```python
from build123d import *

# Parameters (mm, degrees)
SKETCH1_R           = 0.75
SKETCH1_W           = 10.15
SKETCH1_H           = 5.15
BOSS_EXTRUDE1_DEPTH = 7
SKETCH2_W           = 13.15
SKETCH2_H           = 8.15
BOSS_EXTRUDE2_DEPTH = 2


with BuildPart() as part:
    # Sketch1 → Boss-Extrude1 (new body)
    with BuildSketch(Plane.XY):
        with BuildLine():
            Line((-6.58, 4.075), (-1.505, 4.075))
            Line((-1.505, 4.075), (-1.505, 5.575))
            ThreePointArc((-1.505, 5.575), (-0.005, 7.075), (1.495, 5.575))
            Line((1.495, 5.575), (1.495, 4.075))
            Line((1.495, 4.075), (6.57, 4.075))
            Line((6.57, 4.075), (6.57, -4.075))
            Line((6.57, -4.075), (-6.58, -4.075))
            Line((-6.58, -4.075), (-6.58, 4.075))
        make_face()
        with Locations((-0.005, 5.575)):
            Circle(SKETCH1_R, mode=Mode.SUBTRACT)
        with Locations((-0.005, 0)):
            Rectangle(SKETCH1_W, SKETCH1_H, mode=Mode.SUBTRACT)
    extrude(amount=BOSS_EXTRUDE1_DEPTH)

    # Sketch2 → Boss-Extrude2 (add)
    with BuildSketch(Plane.XY.offset(7)):
        with Locations((-0.005, 0)):
            Rectangle(SKETCH2_W, SKETCH2_H)
    extrude(amount=-BOSS_EXTRUDE2_DEPTH)


solid = part.part
```
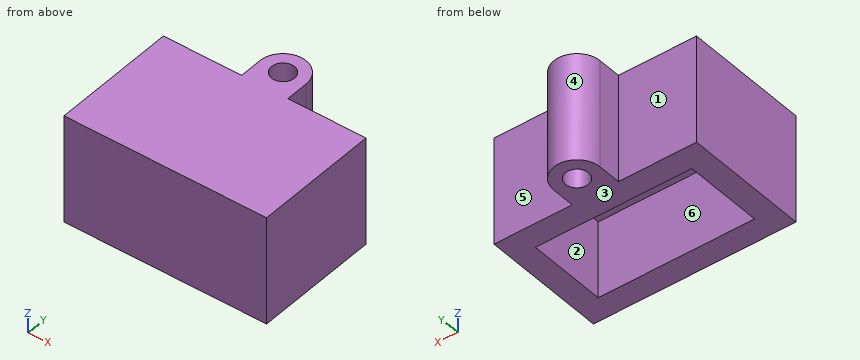
For this review, take the finished solid that the model builds, in its own axes (mm). Face numbers are marked on the shaded views. A direction names the side the tool comes from. Round coordinates to 2 decimals unless told otherwise and drop trailing zeros. Write each loop counter-clockwise with the first axis right and the second up, starting at its lowest first coordinate (ties: lowest second). Pieces come first, ordered by that corner, then holes. Notation, with made-up numbers: (-28, 14) -> (21, 14) arc R6 ccw to (21, 24) -> close; hole circle Ø2 at (31.5, 71). An arc over 180 degrees is marked (long way). One line per question, with ' | ' between items. Start each with the question number.
(1) Mouldability with a two-part tool opening along X and no side actions: class the marked faces 4, 5 and 6 as released by +X, released by -X, zero draft, split by the parting line, or undercut.
(2) Add section D-D, the plane y = -2. Write out the cut boundary in (x, z).
(3) Add section B-B, the plane z = 2.5. Write out the cut boundary in (x, y) (3 decimals), plus the area to 3 significant figures.
(4) Add section A-A, the plane y = 6. Write out the cut boundary in (x, z).
(5) Add section C-C, the plane x = 4.5. Write out the cut boundary in (y, z) (3 decimals), plus the area to 3 significant figures.
(6) Insertion check: P1, Ø1.2, axis at y = 5, z = 4.5, coming from the -X side (3 decimals); P2, Ø2.5, axis at x = -1.5, z = 3.5, coming from the +Y side; P3, Ø4, axis at x = -5, z = 2.5, coming from the +Y side (3 decimals). Each pin has a flat end and moves straight along its axis. Give the tip position at first contact, or say it passes through.
(7) Tool access review of the marked faces 1, 2 and 3: name each direction out of +Z, -Z, +X, -X, +Y, -Y from which nothing blocks a thin tool from reaching the whole face with its end or side.
(8) For line 1 along Y through (x, z) = (0, 1.25) (3 decimals); line 2 along X through (y, z) = (-1.25, 2.25); line 3 along Y through (x, z) = (2.75, 3.25) (3 decimals), list the stretches that pass through material, from the lowest coordinate up. Write a range as from..to.
Answer list:
1) face 4: split by the parting line | face 5: zero draft | face 6: undercut
2) outline: (-6.58, 0) -> (-5.08, 0) -> (-5.08, 5) -> (5.07, 5) -> (5.07, 0) -> (6.57, 0) -> (6.57, 7) -> (-6.58, 7) -> close
3) outline: (-6.58, -4.075) -> (6.57, -4.075) -> (6.57, 4.075) -> (1.495, 4.075) -> (1.495, 5.575) arc R1.5 ccw to (-1.505, 5.575) -> (-1.505, 4.075) -> (-6.58, 4.075) -> close; hole (-5.08, -2.575) -> (5.07, -2.575) -> (5.07, 2.575) -> (-5.08, 2.575) -> close; hole circle Ø1.5 at (-0.005, 5.575) | area: 61.2 mm²
4) outline: (-1.44, 0) -> (-0.62, 0) -> (-0.62, 7) -> (-1.44, 7) -> close; (0.61, 0) -> (1.43, 0) -> (1.43, 7) -> (0.61, 7) -> close
5) outline: (-4.075, 0) -> (-2.575, 0) -> (-2.575, 5) -> (2.575, 5) -> (2.575, 0) -> (4.075, 0) -> (4.075, 7) -> (-4.075, 7) -> close | area: 31.3 mm²
6) P1: x = -1.505 | P2: y = 7.05 | P3: y = 4.075
7) face 1: +Z, -Z, -X, +Y | face 2: -Z | face 3: -Z, +X, -X, +Y, -Y
8) line 1: -4.075..-2.575, 2.575..4.825, 6.325..7.075 | line 2: -6.58..-5.08, 5.07..6.57 | line 3: -4.075..-2.575, 2.575..4.075
